Input: dimensioned drawing with shaded views. Units: mm. Origin: part minimum x, y, z. Coordinates: 2 decimals unless noted, no trailing zeros. Loops run counter-clockwise (first coordinate to the right, second up) from the corner with the lowest first, then second, coordinate; pieces in that order, holes last. Notation, with made-up numbers: (17.5, 65.5) - (60.5, 65.5) arc R36 cw to (60.5, 102.5) - close; hole circle Ø7 at (-2, 15). An arc over 180 degrees is marked (long way). Put each result on its own line as item: value. Start each with the question number.
1) Section C-C on y = 10.5. Output: boundary loops of the cut face in (x, z).
2) Draft query along Y for the marked faces 1, 2, 3 and 4. Return one class per face: +Y half, -Y half, draft (parallel to the pull), parting line (faces both ways), or undercut.
3) Section A-A on z = 1.25. Output: boundary loops of the cut face in (x, y).
4) Section D-D on x = 3. Output: boundary loops of the cut face in (y, z), and give its area (3 significant figures).
5) Contact query for flat-ended pins moving along their axis: pin 1 Ø1 at (x, z) = (2, 2) entering from -Y; pin 2 Ø1 at (x, z) = (1.5, 1) entering from +Y. Output: stop coordinate, or through.
6) Section B-B on y = 8.25. Output: boundary loops of the cut face in (x, z), and give its area (3 significant figures).
7) Material intervals for line 1 along X through (y, z) = (6.25, 5.25) (1 decimal); line 2 along X through (y, z) = (6.5, 2); line 3 along X through (y, z) = (2.5, 4.5), sorted ascending. Write a range as from..to.
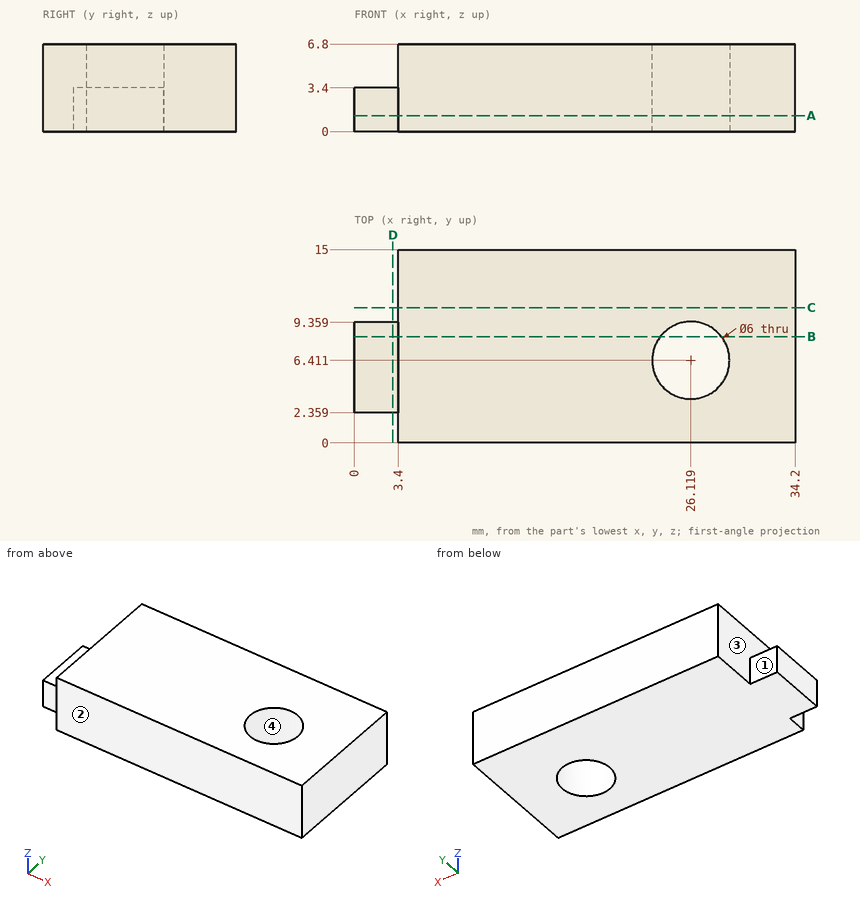
Answer block:
1. outline: (3.4, 0) - (34.2, 0) - (34.2, 6.8) - (3.4, 6.8) - close
2. face 1: +Y half
2. face 2: -Y half
2. face 3: draft
2. face 4: undercut
3. outline: (0, 2.36) - (3.4, 2.36) - (3.4, 0) - (34.2, 0) - (34.2, 15) - (3.4, 15) - (3.4, 9.36) - (0, 9.36) - close; hole circle Ø6 at (26.12, 6.41)
4. outline: (2.36, 0) - (9.36, 0) - (9.36, 3.4) - (2.36, 3.4) - close
4. area: 23.8 mm²
5. pin 1: stops at y = 2.36
5. pin 2: stops at y = 9.36
6. outline: (0, 0) - (23.75, 0) - (23.75, 6.8) - (3.4, 6.8) - (3.4, 3.4) - (0, 3.4) - close; (28.49, 0) - (34.2, 0) - (34.2, 6.8) - (28.49, 6.8) - close
6. area: 189 mm²
7. line 1: x = 3.4..23.1, 29.1..34.2
7. line 2: x = 0..23.12, 29.12..34.2
7. line 3: x = 3.4..34.2
